```python
from build123d import *

# Parameters (mm, degrees)
F0_W     = 135
F0_H     = 200
F1_DEPTH = 4
F2_R     = 1
F4_DEPTH = 6
F5_R     = 1


with BuildPart() as f1:
    # F0 (on Top) → F1 (new body)
    with BuildSketch(Plane.XY):
        with Locations((67.5, 100)):
            Rectangle(F0_W, F0_H)
    extrude(amount=F1_DEPTH)

    # F2
    f2_edges = [f1.edges().sort_by_distance(p)[0] for p in [
        (0, 100, 4),
        (67.5, 0, 4),
        (135, 100, 4),
        (67.5, 200, 4),
        (0, 100, 0),
        (67.5, 0, 0),
        (135, 100, 0),
        (67.5, 200, 0),
        (135, 0, 2),
        (0, 0, 2),
        (135, 200, 2),
        (0, 200, 2),
    ]]
    fillet(f2_edges, radius=F2_R)

    # F3 (on face) → F4 (join)
    with BuildSketch(Plane.XY.offset(4)):
        Polygon((22.5, 167.839746), (30, 172.169873), (30, 180.830127), (22.5, 185.160254), (15, 180.830127), (15, 172.169873), align=None)
        Polygon((120, 180.830127), (112.5, 185.160254), (105, 180.830127), (105, 172.169873), (112.5, 167.839746), (120, 172.169873), align=None)
        Polygon((30, 19.169873), (30, 27.830127), (22.5, 32.160254), (15, 27.830127), (15, 19.169873), (22.5, 14.839746), align=None)
        Polygon((105, 19.169873), (112.5, 14.839746), (120, 19.169873), (120, 27.830127), (112.5, 32.160254), (105, 27.830127), align=None)
    extrude(amount=F4_DEPTH)

    # F5
    f5_edges = [f1.edges().sort_by_distance(p)[0] for p in [
        (18.75, 170.004809, 10),
        (26.25, 170.004809, 10),
        (30, 176.5, 10),
        (26.25, 182.995191, 10),
        (18.75, 182.995191, 10),
        (15, 176.5, 10),
        (120, 176.5, 10),
        (116.25, 182.995191, 10),
        (108.75, 182.995191, 10),
        (105, 176.5, 10),
        (108.75, 170.004809, 10),
        (116.25, 170.004809, 10),
        (108.75, 29.995191, 10),
        (105, 23.5, 10),
        (108.75, 17.004809, 10),
        (116.25, 17.004809, 10),
        (120, 23.5, 10),
        (116.25, 29.995191, 10),
        (26.25, 17.004809, 10),
        (30, 23.5, 10),
        (26.25, 29.995191, 10),
        (18.75, 29.995191, 10),
        (15, 23.5, 10),
        (18.75, 17.004809, 10),
    ]]
    fillet(f5_edges, radius=F5_R)


solid = f1.part
```
Part model, mm, in its own coordinate system. A direction names the side the tool comes from. Round coordinates to 2 decimals unless told otherwise and drop trailing zeros. Loops run counter-clockwise (first coordinate to the right, second up) from the corner with the lowest first, then second, coordinate; pieces in that order, holes last.
Item 1: Drill centre lines: line 1 (X direction, y = 174.5, z = 6.75); line 2 (Y direction, x = 29.5, z = 5.5); line 3 (Z direction, x = 84, y = 79). Where is each one in solid material? Low to high.
Item 2: Cut at A-A, the plane z = 6.5. Give the cut face in (x, y).
Item 3: Cut at B-B, the plane x = 101. Give the cut face in (y, z).
Item 4: Drop flat-ended pins along their axis: P1, Ø1.5, axis at x = 27.5, z = 8, coming from the +Y side; P2, Ø4, axis at y = 24.5, z = 7, coming from the -X side; P3, Ø5.5, axis at y = 175.5, z = 7.5, coming from the +X side; P4, Ø2, axis at y = 144, z = 6.5, coming from the +X side. Give the stop position or say it passes through.
Item 5: 3-axis set-ups, long thin cutter, end or side, ignore diameter. For faces 1 (the face through (18.802, 183.026, 6.465)), 2 (the face through (116.302, 29.965, 6.465)), 3 (the face through (18.698, 170.035, 6.465)): which of +Z, -Z, +X, -X, +Y, -Y reach the whole face in a straight line?
Item 6: Cut at C-C, the plane y = 152. Give the cut face in (x, z), then the cut area to 3 significant figures.
Item 7: Mould opens along Y. For faces 4 (the face through (26.16, 17.28, 9.7)), 5 (the face through (26.198, 169.974, 6.465)), 6 (the face through (120, 23, 6)), 7 (the face through (116.16, 170.28, 9.7)) say: +Y half, -Y half, draft (parallel to the pull), parting line (faces both ways), or undercut.
A:
1. line 1: x = 15 to 30, 105 to 120
1. line 2: y = 18.88 to 28.12, 171.88 to 181.12
1. line 3: z = 0 to 4
2. outline: (15, 19.17) - (22.5, 14.84) - (30, 19.17) - (30, 27.83) - (22.5, 32.16) - (15, 27.83) - close; (15, 172.17) - (22.5, 167.84) - (30, 172.17) - (30, 180.83) - (22.5, 185.16) - (15, 180.83) - close; (105, 19.17) - (112.5, 14.84) - (120, 19.17) - (120, 27.83) - (112.5, 32.16) - (105, 27.83) - close; (105, 172.17) - (112.5, 167.84) - (120, 172.17) - (120, 180.83) - (112.5, 185.16) - (105, 180.83) - close
3. outline: (0, 1) arc R1 ccw to (1, 0) - (199, 0) arc R1 ccw to (200, 1) - (200, 3) arc R1 ccw to (199, 4) - (1, 4) arc R1 ccw to (0, 3) - close
4. P1: stops at y = 182.71
4. P2: stops at x = 15
4. P3: stops at x = 120
4. P4: passes through
5. face 1: +Z, -X, +Y
5. face 2: +Z, +X
5. face 3: +Z, -X
6. outline: (0, 1) arc R1 ccw to (1, 0) - (134, 0) arc R1 ccw to (135, 1) - (135, 3) arc R1 ccw to (134, 4) - (1, 4) arc R1 ccw to (0, 3) - close
6. area: 539 mm2
7. face 4: -Y half
7. face 5: undercut
7. face 6: draft
7. face 7: undercut
